from build123d import *

# Parameters (mm, degrees)
SKETCH1_R                     = 14.605
BOSS_EXTRUDE2_DEPTH           = 25.4
SKETCH10_R                    = 5.715
CUT_EXTRUDE5_DEPTH            = 48.424233935
SKETCH11_R                    = 6.6675
CUT_EXTRUDE6_DEPTH            = 1.27
SKETCH12_OUTSIDE_W            = 40.908
SKETCH12_OUTSIDE_H            = 40.908
SKETCH12_OUTSIDE_R            = 10.414
CUT_EXTRUDE7_DEPTH            = 17.78
CIRPATTERN1_COUNT             = 3
CIRPATTERN2_COUNT             = 2
SKETCH26_R                    = 1.651
CUT_EXTRUDE8_DEPTH            = 8.89
CIRPATTERN3_COUNT             = 2
SKETCH27_R                    = 0.79375
CUT_EXTRUDE9_DEPTH            = 24.13
TAP_DRILL_FOR_0_80_TAP3_D     = 1.19126
TAP_DRILL_FOR_0_80_TAP3_DEPTH = 6.35
TAP_DRILL_FOR_0_80_TAP3_TIP   = 0.499792913
CUT_EXTRUDE10_START           = 15.24
SKETCH33_R                    = 10.414
SKETCH33_R_2                  = 9.7028
CUT_EXTRUDE10_DEPTH           = 15.24
BOSS_EXTRUDE3_START           = 2.54
SKETCH33_2_R                  = 10.414
SKETCH33_2_R_2                = 9.7028
BOSS_EXTRUDE3_DEPTH           = 2.54
SKETCH35_R                    = 0.7112
CUT_EXTRUDE11_DEPTH           = 3.556


with BuildPart() as part:
    # Sketch1 → Boss-Extrude2 (new body)
    with BuildSketch(Plane(origin=(0, 0, 0), x_dir=(1, 0, 0), z_dir=(0, 1, 0))):
        with Locations(Location((13.028153923, -14.383045271, 0), (0, 0, 270))):
            Circle(SKETCH1_R)
    extrude(amount=BOSS_EXTRUDE2_DEPTH)

    # Sketch10 → Cut-Extrude5 (cut, through all)
    with BuildSketch(Plane(origin=(0, 25.4, 0), x_dir=(1, 0, 0), z_dir=(0, 1, 0))):
        with Locations(Location((13.028153923, -14.383045271, 0), (0, 0, 270))):
            Circle(SKETCH10_R)
    extrude(amount=-CUT_EXTRUDE5_DEPTH, mode=Mode.SUBTRACT)

    # Sketch11 → Cut-Extrude6 (cut)
    with BuildSketch(Plane(origin=(0, 25.4, 0), x_dir=(1, 0, 0), z_dir=(0, 1, 0))):
        with Locations(Location((13.028153923, -14.383045271, 0), (0, 0, 270))):
            Circle(SKETCH11_R)
    extrude(amount=-CUT_EXTRUDE6_DEPTH, mode=Mode.SUBTRACT)

    # Sketch12 outside → Cut-Extrude7 (cut)
    with BuildSketch(Plane(origin=(0, 25.4, 0), x_dir=(1, 0, 0), z_dir=(0, 1, 0))):
        with Locations((13.028, -14.383)):
            Rectangle(SKETCH12_OUTSIDE_W, SKETCH12_OUTSIDE_H)
        with Locations(Location((13.028153923, -14.383045271, 0), (0, 0, 270))):
            Circle(SKETCH12_OUTSIDE_R, mode=Mode.SUBTRACT)
    extrude(amount=-CUT_EXTRUDE7_DEPTH, mode=Mode.SUBTRACT)

    # Sketch17 → 50 _0.07_ Diameter Hole1 (revolve, cut)
    with BuildSketch(Plane(origin=(4.692367215, 25.4, 13.504077717), x_dir=(0, 0, 1), z_dir=(1, 0, 0))):
        Polygon((0, 0), (0, 3.07416509), (0.889, 2.54), (0.889, 0), align=None)
    f_50_0_07_diameter_hole1 = revolve(axis=Axis((4.692367215, 31.75, 13.504077717), (0, -1, 0)), mode=Mode.SUBTRACT)

    # CirPattern1: 50 _0.07_ Diameter Hole1 ×3 about axis
    cirpattern1_axis = Axis((13.028153923, 0, 14.383045271), (0, 1, 0))
    for i in range(1, CIRPATTERN1_COUNT):
        add(f_50_0_07_diameter_hole1.rotate(cirpattern1_axis, i * 360 / CIRPATTERN1_COUNT), mode=Mode.SUBTRACT)

    # Sketch24 → 1_16 _0.0625_ Diameter Hole2 (revolve, cut)
    with BuildSketch(Plane(origin=(8.163266455, 0, 24.388191195), x_dir=(0, 0, -1), z_dir=(1, 0, 0))):
        Polygon((0, 0), (0, 4.477433116), (0.79375, 4.0005), (0.79375, 0), align=None)
    f_1_16_0_0625_diameter_hole2 = revolve(axis=Axis((8.163266455, -6.35, 24.388191195), (0, 1, 0)), mode=Mode.SUBTRACT)

    # CirPattern2: 1_16 _0.0625_ Diameter Hole2 ×2 about axis
    cirpattern2_axis = Axis((13.028153923, 0, 14.383045271), (0, 1, 0))
    for i in range(1, CIRPATTERN2_COUNT):
        add(f_1_16_0_0625_diameter_hole2.rotate(cirpattern2_axis, i * 360 / CIRPATTERN2_COUNT), mode=Mode.SUBTRACT)

    # Sketch26 → Cut-Extrude8 (cut)
    with BuildSketch(Plane(origin=(0, 0, 0), x_dir=(-1, 0, 0), z_dir=(0, -1, 0))):
        with Locations(Location((-1.606754466, -8.829520764, 0), (0, 0, 90))):
            Circle(SKETCH26_R)
    cut_extrude8 = extrude(amount=-CUT_EXTRUDE8_DEPTH, mode=Mode.SUBTRACT)

    # CirPattern3: Cut-Extrude8 ×2 about axis
    cirpattern3_axis = Axis((13.028153923, 0, 14.383045271), (0, 1, 0))
    for i in range(1, CIRPATTERN3_COUNT):
        add(cut_extrude8.rotate(cirpattern3_axis, i * 360 / CIRPATTERN3_COUNT), mode=Mode.SUBTRACT)

    # Sketch27 → Cut-Extrude9 (cut)
    with BuildSketch(Plane(origin=(0, 0, 0), x_dir=(-1, 0, 0), z_dir=(0, -1, 0))):
        with Locations(Location((-5.827402564, -17.142659866, 0), (0, 0, 90))):
            Circle(SKETCH27_R)
    extrude(amount=-CUT_EXTRUDE9_DEPTH, mode=Mode.SUBTRACT)

    # Tap Drill for _0-80 Tap3
    with Locations(Plane(origin=(0, 0, 0), x_dir=(-1, 0, 0), z_dir=(0, -1, 0))):
        with Locations((-5.827402564, -15.237659866), (-5.827402564, -19.047659866)):
            Hole(TAP_DRILL_FOR_0_80_TAP3_D / 2, depth=TAP_DRILL_FOR_0_80_TAP3_DEPTH)
            with Locations((0, 0, -(TAP_DRILL_FOR_0_80_TAP3_DEPTH + TAP_DRILL_FOR_0_80_TAP3_TIP / 2))):  # 100° drill point
                Cone(0, TAP_DRILL_FOR_0_80_TAP3_D / 2, TAP_DRILL_FOR_0_80_TAP3_TIP, mode=Mode.SUBTRACT)

    # Sketch33 → Cut-Extrude10 (cut)
    with BuildSketch(Plane(origin=(0, 7.62, 0), x_dir=(1, 0, 0), z_dir=(0, 1, 0)).offset(CUT_EXTRUDE10_START)):
        with Locations(Location((13.028153923, -14.383045271, 0), (0, 0, 270))):
            Circle(SKETCH33_R)
        with Locations(Location((13.028153923, -14.383045271, 0), (0, 0, 90))):
            Circle(SKETCH33_R_2, mode=Mode.SUBTRACT)
    extrude(amount=-CUT_EXTRUDE10_DEPTH, mode=Mode.SUBTRACT)

    # Sketch33_2 → Boss-Extrude3 (add)
    with BuildSketch(Plane(origin=(0, 7.62, 0), x_dir=(1, 0, 0), z_dir=(0, 1, 0)).offset(BOSS_EXTRUDE3_START)):
        with Locations(Location((13.028153923, -14.383045271, 0), (0, 0, 270))):
            Circle(SKETCH33_2_R)
        with Locations(Location((13.028153923, -14.383045271, 0), (0, 0, 90))):
            Circle(SKETCH33_2_R_2, mode=Mode.SUBTRACT)
    extrude(amount=-BOSS_EXTRUDE3_DEPTH)

    # Sketch35 → Cut-Extrude11 (cut)
    with BuildSketch(Plane(origin=(0, 25.4, 0), x_dir=(1, 0, 0), z_dir=(0, 1, 0))):
        with Locations((22.490332014, -18.732594877)):
            Circle(SKETCH35_R)
    extrude(amount=-CUT_EXTRUDE11_DEPTH, mode=Mode.SUBTRACT)


solid = part.part
Design review of the part built by this model. Coordinates are the model's own, in mm. A direction names the side the tool comes from. Give positions to 0.01 mm unless a question says otherwise; leave off trailing zeros. Write each loop counter-clockwise with the first axis right and the second up, starting at its lowest first coordinate (ties: lowest second). Pieces come first, ordered by that corner, then holes. Notation, with made-up numbers: M -13.5,80.25 L 6.5,80.25 A37 ccw 6.5,117.25 Z; hole C 82,89.25 d10. An arc over 180 degrees is marked long. Answer as a JSON object with one key per item and string values. Group by question number.
1) We need section C-C (y = 23.25). Give the boundary of the cut face in (x, z) (1 decimal).
2) Mouldability with a two-part tool opening along X and no side actions: class faces 1 (the face through (12.602, 16.599, 24.076)), 2 (the face through (5.85, 6.76, 15.34)), 3 (the face through (6, 24.13, 17)), 4 (the face through (22, 10.16, 10)) as released by +X, released by -X, zero draft, split by the parting line, or undercut.
3) We need section A-A (x = 9.75). Give the boundary of the cut face in (y, z).
4) For line 1 along Y through (x, z) = (26.5, 10.25); line 2 along X through (y, z) = (9.5, 11); line 3 along X through (y, z) = (19.5, 13.5), list the stretches that pass through material, from the lowest coordinate up.
5) Tool access review of faces 5 (the face through (8.6, 7.62, 24.1)), 6 (the face through (5.862, 11.896, 17.936)), 7 (the face through (13, 0, 21)), 8 (the face through (6, 22.86, 7)), 9 (the face through (13.2, 25.4, 21.2)): name each direction out of +Z, -Z, +X, -X, +Y, -Y from which nothing blocks a thin tool from reaching the whole face with its end or side.
6) We need section B-B (z = 11). Give the boundary of the cut face in (x, y), and give its area (3 significant figures).
7) Clearance check with flat-ended pins moving along their axes: pin 1 Ø1.4 at (x, z) = (8.16, 24.39) entering from -Y; pin 2 Ø10 at (x, z) = (9.5, 18.5) entering from -Y; pin 3 Ø1.5 at (y, z) = (17.5, 12) entering from +X; pin 4 Ø1.5 at (y, z) = (8.5, 14) entering from -X. State where each tip first meets the part, or that it passes through.
8) We need section D-D (y = 16). Give the boundary of the cut face in (x, z) (1 decimal), and give its area (3 significant figures).
Answer key:
{
 "1": {"outline": "M 22.2,19.4 A10.4 ccw long 22.8,18.1 A0.7 cw Z; hole C 4.7,13.5 d1.8; hole C 5.8,17.1 d1.6; hole C 13,14.4 d11.4; hole C 16.4,22 d1.8; hole C 18,7.6 d1.8"},
 "2": {"face 1": "split by the parting line", "face 2": "undercut", "face 3": "undercut", "face 4": "zero draft"},
 "3": {"outline": "M 0,0.15 L 7.62,0.15 L 7.62,4.5 L 10.16,4.5 L 10.16,5.25 L 22.86,5.25 L 22.86,4.5 L 25.4,4.5 L 25.4,8.58 L 24.13,8.58 L 24.13,9.7 L 0,9.7 Z; M 0,19.06 L 24.13,19.06 L 24.13,20.19 L 25.4,20.19 L 25.4,24.27 L 22.86,24.27 L 22.86,23.52 L 10.16,23.52 L 10.16,24.27 L 7.62,24.27 L 7.62,28.62 L 0,28.62 Z"},
 "4": {"line 1": "y = 0 to 7.62", "line 2": "x = 3.18 to 8.42, 17.63 to 22.88", "line 3": "x = 3.37 to 7.38, 18.67 to 22.69"},
 "5": {"face 5": "+Y", "face 6": "-Y", "face 7": "+Z, -Z, +X, -X, -Y", "face 8": "none", "face 9": "+Z, -Z, +X, -X, +Y"},
 "6": {"outline": "M -1.18,0 L 8.42,0 L 8.42,24.13 L 7.28,24.13 L 7.28,25.4 L 3.18,25.4 L 3.18,22.86 L 3.93,22.86 L 3.93,10.16 L 3.18,10.16 L 3.18,7.62 L -1.18,7.62 Z; M 17.63,0 L 27.24,0 L 27.24,7.62 L 22.88,7.62 L 22.88,10.16 L 22.12,10.16 L 22.12,22.86 L 22.88,22.86 L 22.88,25.4 L 18.77,25.4 L 18.77,24.13 L 17.63,24.13 Z", "area": "311 mm²"},
 "7": {"pin 1": "stops at y = 4.05", "pin 2": "stops at y = 0", "pin 3": "stops at x = 22.59", "pin 4": "stops at x = 2.61"},
 "8": {"outline": "C 13,14.4 d19.4; hole C 5.8,17.1 d1.6; hole C 13,14.4 d11.4", "area": "191 mm²"}
}
